CAD build for the part. Positions are in the model's coordinates, mm. A direction names the side the tool comes from. Coordinates: 2 decimals unless noted, no trailing zeros. Write each loop counter-clockwise with the first axis right and the second up, starting at its lowest first coordinate (ties: lowest second). Pieces come first, ordered by that corner, then holes.
```python
from build123d import *

# Parameters (mm, degrees)
SKETCH_1_R          = 2
EXTRUDE_1_DEPTH     = 32
SKETCH_2_R          = 3.5
EXTRUDE_2_DEPTH     = 2
FILLET_1_R          = 1
CUT_EXTRUDE_1_DEPTH = 2


with BuildPart() as part:
    # 草图1 → 凸台-拉伸1 (new body)
    with BuildSketch(Plane.XY):
        Circle(SKETCH_1_R)
    extrude(amount=EXTRUDE_1_DEPTH)

    # 草图2 → 凸台-拉伸2 (add)
    with BuildSketch(Plane.XY.offset(32)):
        Circle(SKETCH_2_R)
    extrude(amount=EXTRUDE_2_DEPTH)

    # 圆角1
    fillet_1_edges = [part.edges().sort_by_distance(p)[0] for p in [
        (-3.5, 0, 34),
    ]]
    fillet(fillet_1_edges, radius=FILLET_1_R)

    # 草图3 → 切除-拉伸1 (cut)
    with BuildSketch(Plane.XY.offset(34)):
        Polygon((0, 1.5), (0.5, 1.5), (0.5, 0.5), (1.5, 0.5), (1.5, -0.5), (0.5, -0.5), (0.5, -1.5), (-0.5, -1.5), (-0.5, -0.5), (-1.5, -0.5), (-1.5, 0.5), (-0.5, 0.5), (-0.5, 1.5), align=None)
    extrude(amount=-CUT_EXTRUDE_1_DEPTH, mode=Mode.SUBTRACT)


solid = part.part
```
Item 1: Wall check: line 1 along Z through (x, y) = (-1.75, 1.25); line 2 along Y through (x, z) = (-0.25, 6.5); line 3 along Y through (x, z) = (-1.75, 14.5). Give the ranges that are in metal, low to high.
Item 2: Two-plate mould, pull along X, no slides. Class faces 4 (the flat face through (0, 0, 0)), 5 (the cylindrical face through (3.233, -1.341, 32.493)), 6 (the flat face through (0, -1.5, 33)): +X half, -X half, draft (parallel to the pull), parting line (faces both ways), or undercut.
Item 3: Saw through at A-A, the plane y = 0. Write the cut outline in (x, z).
Item 4: Which spindle directions (+Z, -Z, +X, -X, +Y, -Y) get a long thin tool onto all of the face, cutting with end or side? Do faces 1 (the flat face through (2, -2, 32)), 2 (the flat face through (1, -1, 34)), 3 (the flat face through (0, 1.5, 33)). Say none if no direction does.
Item 5: Saw through at C-C, the plane z = 5. Write the cut outline in (x, y), and give its area (3 significant figures).
Item 6: Flat gauge pins, fed straight in: pin 1 Ø0.8 at (x, z) = (-1, 33) entering from +Y; pin 2 Ø1 at (y, z) = (1.5, 26.5) entering from +X; pin 3 Ø3 at (x, z) = (-0.5, 21) entering from +Y. Where does each tip first touch, or does it go through?
Working result:
1. line 1: z = 32 to 34
1. line 2: y = -1.98 to 1.98
1. line 3: y = -0.97 to 0.97
2. face 4: draft
2. face 5: parting line
2. face 6: undercut
3. outline: (-3.5, 32) - (-2, 32) - (-2, 0) - (2, 0) - (2, 32) - (3.5, 32) - (3.5, 33) arc R1 ccw to (2.5, 34) - (1.5, 34) - (1.5, 32) - (-1.5, 32) - (-1.5, 34) - (-2.5, 34) arc R1 ccw to (-3.5, 33) - close
4. face 1: -Z
4. face 2: +Z, +X, -X, +Y, -Y
4. face 3: +Z
5. outline: circle Ø4 at (0, 0)
5. area: 12.6 mm2
6. pin 1: stops at y = 3.45
6. pin 2: stops at x = 1.73
6. pin 3: stops at y = 2
